The drawing under review shows one solid part. Ordinate dimensions are in mm from its lowest x, y, z. Give positions to 0.01 mm unless a question says otherwise; leave off trailing zeros. Loops run counter-clockwise (first coordinate to the right, second up) from the corner with the lowest first, then second, coordinate; pieces in that order, holes last. Notation, with made-up numbers: (45.25, -35.75) - (87.25, -35.75) arc R19 ccw to (87.25, -3.75) - close; hole circle Ø6 at (-33.75, 89). An arc over 180 degrees is marked (long way). Answer as CSV lines item,"result".
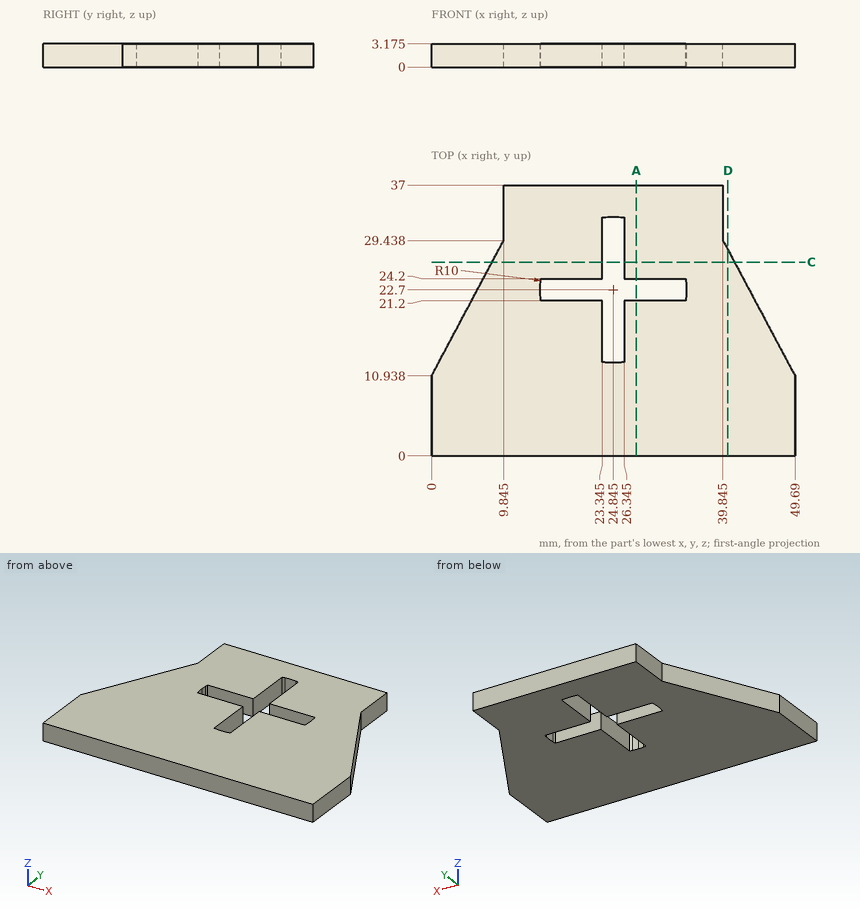
1) Wall thickness on line 1 (Y direction, x = 30, z = 2.95); line 2 (X direction, y = 30, z = 1.2) (1 decimal); line 3 (X direction, y = 33.5, z = 0.95) (1 decimal): over which ranges is each line inside the solid? List them lowest first. Write a range as from..to.
From the geometry:
line 1,"y = 0..21.2, 24.2..37"
line 2,"x = 9.8..23.3, 26.3..39.8"
line 3,"x = 9.8..39.8"
2) Insertion check: P1, Ø1.5, axis at y = 32, z = 0.5, coming from the -X side (1 decimal); P2, Ø1, axis at x = 42, z = 1.5, coming from the +Y side (1 decimal); P3, Ø1, axis at y = 15, z = 1, coming from the -X side (1 decimal). Each pin has a flat end and moves straight along its axis. Give the tip position at first contact, or say it passes through.
From the geometry:
P1,"stops at x = 9.8"
P2,"stops at y = 26.3"
P3,"stops at x = 1.9"
3) Consider section A-A on x = 28. Write out the cut boundary in (y, z) (1 decimal), and give its area (3 significant figures).
From the geometry:
outline,"(0, 0) - (21.2, 0) - (21.2, 3.2) - (0, 3.2) - close; (24.2, 0) - (37, 0) - (37, 3.2) - (24.2, 3.2) - close"
area,"108 mm^2"
4) Consider section C-C on y = 26.5. Write out the cut boundary in (x, z) (1 decimal).
From the geometry:
outline,"(8.3, 0) - (23.3, 0) - (23.3, 3.2) - (8.3, 3.2) - close; (26.3, 0) - (41.4, 0) - (41.4, 3.2) - (26.3, 3.2) - close"
5) Consider section D-D on x = 40.5. Write out the cut boundary in (y, z) (1 decimal).
From the geometry:
outline,"(0, 0) - (28.2, 0) - (28.2, 3.2) - (0, 3.2) - close"
